Autodesk Inventor part; units mm, degrees
ref_plane "YZ Plane" through (0, 0, 0) normal (1, 0, 0) x (0, 1, 0)
ref_plane "XZ Plane" through (0, 0, 0) normal (0, 1, 0) x (-1, 0, 0)
ref_plane "XY Plane" through (0, 0, 0) normal (0, 0, 1) x (1, 0, 0)
sketch "Sketch1" plane through (0, 0, 0) normal (0, 0, 1) x (1, 0, 0)
  line L0 (0, 0) -> (25.4, 0)
  line L1 (25.4, 0) -> (25.4, 25.4)
  line L2 (25.4, 25.4) -> (0, 25.4)
  line L3 (0, 25.4) -> (0, 0)
  line L4 (1.5875, 23.8125) -> (23.8125, 23.8125)
  line L5 (23.8125, 23.8125) -> (23.8125, 1.5875)
  line L6 (23.8125, 1.5875) -> (1.5875, 1.5875)
  line L7 (1.5875, 1.5875) -> (1.5875, 23.8125)
  dimension "d0" = 25.4
  dimension "d2" = 25.4
  dimension "d3" = 1.5875
extrude "Extrusion1" add sketch "Sketch1" along normal blind 596.9
sketch "Sketch3" plane through (0, 0, 0) normal (0, -1, 0) x (1, 0, 0)
  circle A0 centre (12.7, 574.675) radius 3.3782
  circle A1 centre (12.7, 542.925) radius 3.3782
  circle A2 centre (12.7, 19.05) radius 3.302
  circle A3 centre (12.7, 38.1) radius 3.302
  arc A4 (3.175, 50.8) -> (0, 47.625) centre (3.175, 47.625) ccw
  line L0 (3.175, 50.8) -> (22.225, 50.8)
  arc A5 (25.4, 47.625) -> (22.225, 50.8) centre (22.225, 47.625) ccw
  line L1 (25.4, 47.625) -> (25.4, 4.445)
  line L2 (25.4, 4.445) -> (0, 4.445)
  line L3 (0, 47.625) -> (0, 4.445)
  circle A6 centre (12.7, 431.8) radius 3.3782
  circle A7 centre (12.7, 381) radius 3.3782
  circle A8 centre (12.7, 285.75) radius 3.3782
extrude "Extrusion3" cut sketch "Sketch3" against normal blind 25.4 contours A0 | A1 | A2 | A3 | A6 | A7 | A8
sketch "Sketch4" plane through (0, 0, 0) normal (-1, 0, 0) x (0, 0, 1)
  circle A0 centre (533.4, 12.7) radius 3.3782
  circle A1 centre (584.2, 12.7) radius 3.3782
  line L0 (0, 25.4) -> (0, 0)
  line L1 (596.9, 25.4) -> (596.9, 0)
  line L2 (596.9, 12.7) -> (0, 12.7) construction
  circle A2 centre (501.65, 12.7) radius 3.3782
  circle A3 centre (311.15, 12.7) radius 3.3782
  circle A4 centre (120.65, 12.7) radius 3.3782
  dimension "d12" = 31.75
  dimension "d15" = 190.5
extrude "Extrusion4" cut sketch "Sketch4" against normal blind 25.4
properties part number "Rebuild Edge Mount 4" material "Aluminum 6061"
The model under review builds one solid part; all positions refer to its coordinate system, in mm. A direction names the side the tool comes from. Coordinates: 2 decimals unless noted, no trailing zeros. Write each loop counter-clockwise with the first axis right and the second up, starting at its lowest first coordinate (ties: lowest second). Pieces come first, ordered by that corner, then holes. Notation, with made-up numbers: (42, -33) - (91, -33) arc R22 ccw to (91, 4) - close; hole circle Ø4 at (32, 34.25). An arc over 180 degrees is marked (long way). Answer in a Markdown table with one row per item. Add a question column.
Q1. Clearance check with flat-ended pins moving along their axes: pin 1 (10 mm diameter, centred on x = 3.5, y = 6, fed in from -Z); pin 2 (4 mm diameter, centred on x = 12.7, z = 381, fed in from +Y). State where each tip first meets the part, or that it passes through.
Q2. Draft analysis for pull direction X (two halves, no side actions). For faces 3 (the face through (13, 1.588, 294)), 4 (the face through (25.4, 13, 294)), 5 (the face through (0, 13, 294)), 6 (the face through (1, 13, 0)), state which applies: +X half, -X half, draft (parallel to the pull), parting line (faces both ways), or undercut.
Q3. To check wall thickness, follow line 1 along X through (y, z) = (22.5, 516); line 2 along X through (y, z) = (24.7, 381). State the ranges of each line that lie inside material, in increasing order. Write a range as from..to.
Q4. For faces 1 (the face through (1, 13, 596.9)), 2 (the face through (1.588, 13, 294)), list the 3-axis set-ups (+Z, -Z, +X, -X, +Y, -Y) from which the entire face can be reached by the end or side of a thin tool; tool diameter is ignored.
Q5. Consider section A-A on z = 422.5. Give the boundary of the cut face in (x, y).
Answers below:
| question | item | result |
|---|---|---|
| 1 | pin 1 | z = 0 |
| 1 | pin 2 | through |
| 2 | face 3 | undercut |
| 2 | face 4 | +X half |
| 2 | face 5 | -X half |
| 2 | face 6 | draft |
| 3 | line 1 | 0..1.59, 23.81..25.4 |
| 3 | line 2 | 0..9.32, 16.08..25.4 |
| 4 | face 1 | +Z, +X, -X, +Y, -Y |
| 4 | face 2 | +Z, -Z |
| 5 | outline | (0, 0) - (25.4, 0) - (25.4, 25.4) - (0, 25.4) - close; hole (1.59, 1.59) - (23.81, 1.59) - (23.81, 23.81) - (1.59, 23.81) - close |
